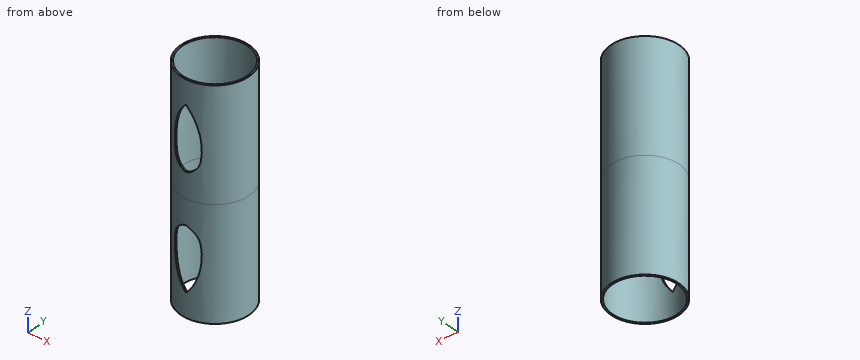
from build123d import *

# Parameters (mm, degrees)
F0_R     = 20
F0_R_2   = 19
F1_DEPTH = 65
F3_DEPTH = 41.1


with BuildPart() as f1:
    # F0 (on Top) → F1 (new body)
    with BuildSketch(Plane.XY):
        Circle(F0_R)
        Circle(F0_R_2, mode=Mode.SUBTRACT)
    extrude(amount=F1_DEPTH)

    # F2 (on Front) → F3 (cut)
    with BuildSketch(Plane.XZ):
        with BuildLine():
            add(Edge.make_bspline(
                [(0, 14.5592805974), (-1.9073922383, 14.7213677243), (-6.1064946547, 17.7360926743), (-8.1839165851, 23.2066328676), (-8.391246048, 36.0351621809), (-3.8296298891, 47.432605238), (-1.2185013376, 49.7799145352), (0, 51.348935332)],
                knots=[0, 0, 0, 0, 0.1765278414, 0.3445091773, 0.5954474838, 0.8373921793, 1, 1, 1, 1], degree=3))
            add(Edge.make_bspline(
                [(0, 14.5592805974), (1.9073922383, 14.7213677243), (6.1064946547, 17.7360926743), (8.1839165851, 23.2066328676), (8.391246048, 36.0351621809), (3.8296298891, 47.432605238), (1.2185013376, 49.7799145352), (0, 51.348935332)],
                knots=[0, 0, 0, 0, 0.1765278414, 0.3445091773, 0.5954474838, 0.8373921793, 1, 1, 1, 1], degree=3))
        make_face()
    extrude(amount=F3_DEPTH, mode=Mode.SUBTRACT)

    # F4: F1 across plane


with BuildPart() as f1_1:
    add(f1.part)
    add(f1.part.mirror(Plane.XY))


solid = f1_1.part
Read the model definition and answer for the solid it produces. Units are mm, in the model's axes. Give positions to 0.01 mm unless a question says otherwise; leave off trailing zeros. Write each loop counter-clockwise with the first axis right and the second up, starting at its lowest first coordinate (ties: lowest second). Pieces come first, ordered by that corner, then holes. Notation, with made-up numbers: (-18, -29.75) - (15, -29.75) arc R8 ccw to (15, -19.75) - close; hole circle Ø1 at (-24.5, 72.25). An arc over 180 degrees is marked (long way). Answer in a Markdown table with one row per item. Add a question column.
Item 1: Section B-B, the plane x = -13 is taken. Write down the section's boundary in (y, z), and give its area (3 significant figures).
Item 2: Section C-C, the plane z = 6 is taken. Write down the section's boundary in (x, y).
Item 3: Flat-ended cylindrical pins translate along their axes: P1, Ø3, axis at x = 9.5, z = 36, coming from the -Y side; P2, Ø10, axis at x = -1.5, z = 10.5, coming from the +Y side; P3, Ø10, axis at y = -11.5, z = -50.5, coming from the -X side; P4, Ø5, axis at x = 10, y = 12.5, coming from the -Z side. Find the tip coordinate at first contact, or state that the pin passes through.
Item 4: Section D-D, the plane x = -3 is taken. Count the separate pieces of the cut face and the enclosed holes in it, and give its area (3 significant figures).
Item 5: Find the intervals of material crossed by L1, parallel to X at y = -0.5, z = 26; L2, parallel to Y at x = 0, z = -23; L3, parallel to X at y = -12.5, z = -52, in increasing order.
Item 6: Section A-A, the plane y = 0 is taken. Write down the section's boundary in (x, z), and give its area (3 significant figures).
Recorded:
| question | item | result |
|---|---|---|
| 1 | outline | (-15.2, -65) - (-13.86, -65) - (-13.86, 65) - (-15.2, 65) - close; (13.86, -65) - (15.2, -65) - (15.2, 65) - (13.86, 65) - close |
| 1 | area | 349 mm2 |
| 2 | outline | circle Ø40 at (0, 0); hole circle Ø38 at (0, 0) |
| 3 | P1 | stops at y = -18.33 |
| 3 | P2 | stops at y = 20 |
| 3 | P3 | stops at x = -18.91 |
| 3 | P4 | passes through |
| 4 | separate pieces | 4 |
| 4 | enclosed holes | 0 |
| 4 | area | 198 mm2 |
| 5 | L1 | x = -19.99 to -18.99, 18.99 to 19.99 |
| 5 | L2 | y = 19 to 20 |
| 5 | L3 | x = -15.61 to -14.31, 14.31 to 15.61 |
| 6 | outline | (-20, -65) - (-19, -65) - (-19, 65) - (-20, 65) - close; (19, -65) - (20, -65) - (20, 65) - (19, 65) - close |
| 6 | area | 260 mm2 |
